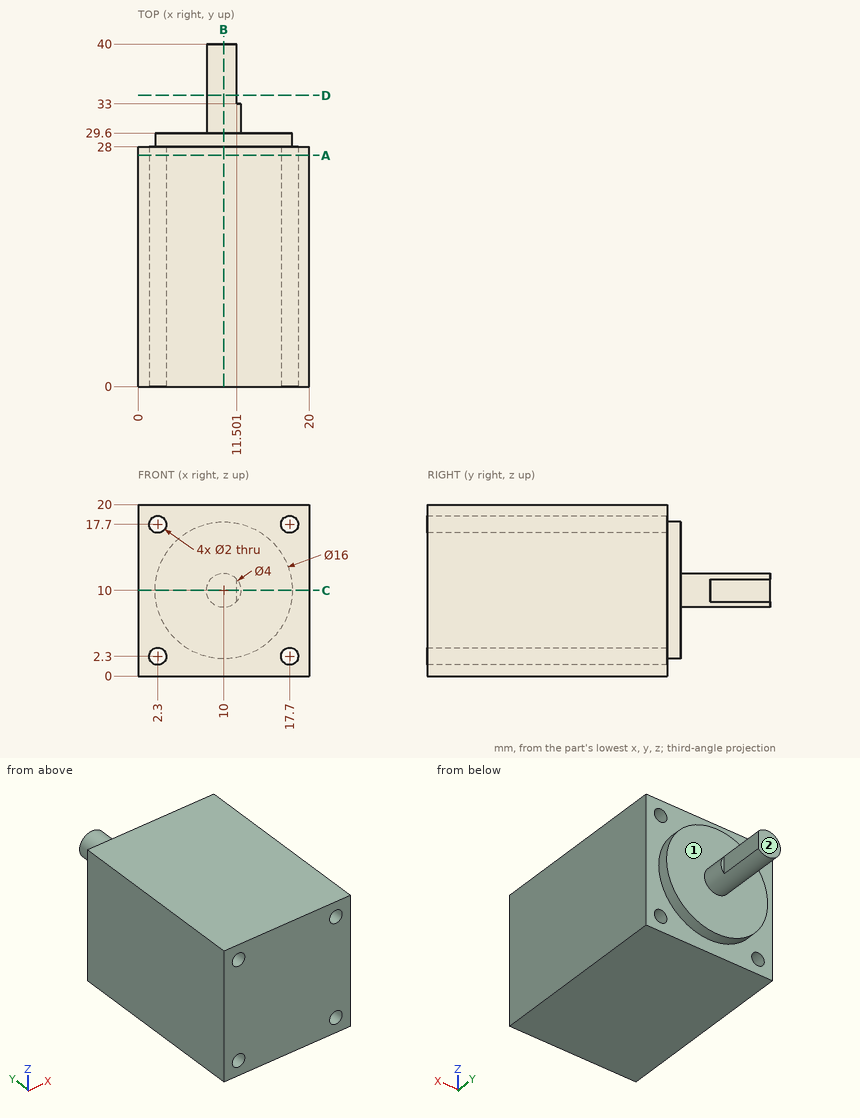
Answer from the drawing. Dimensions are ordinates in mm from the lowest x, y and z of the part. A direction names the side the tool comes from. Give positions to 0.01 mm unless a question says otherwise; leave off trailing zeros. Write each loop counter-clockwise with the first axis right and the second up, starting at its lowest first coordinate (ties: lowest second). Pieces come first, ordered by that corner, then holes. Notation, with made-up numbers: (72.25, 18) -> (95.25, 18) arc R11 cw to (95.25, 27) -> close; hole circle Ø6 at (-25, 42). An arc over 180 degrees is marked (long way). Use a Markdown table: item, result.
(1) Find the intervals of material crossed by probe 1 along X at (y, z) = (13.25, 2.3); probe 2 along Z at (x, y) = (17.25, 3.5); probe 3 along Y at (x, z) = (5.5, 17), in increasing order. Write a range as from..to.
Return value:
| item | result |
|---|---|
| probe 1 | 0..1.3, 3.3..16.7, 18.7..20 |
| probe 2 | 0..1.41, 3.19..16.81, 18.59..20 |
| probe 3 | 0..28 |
(2) Section A-A, the plane y = 27 is taken. Determine the outline of the cut face in (x, z), then the cut area to 3 significant figures.
Return value:
| item | result |
|---|---|
| outline | (0, 0) -> (20, 0) -> (20, 20) -> (0, 20) -> close; hole circle Ø2 at (2.3, 2.3); hole circle Ø2 at (2.3, 17.7); hole circle Ø2 at (17.7, 2.3); hole circle Ø2 at (17.7, 17.7) |
| area | 387 mm2 |
(3) Section D-D, the plane y = 34 is taken. Determine the outline of the cut face in (x, z), then the cut area to 3 significant figures.
Return value:
| item | result |
|---|---|
| outline | (11.5, 8.68) -> (11.5, 11.32) arc R2 ccw (long way) to start |
| area | 11.7 mm2 |
(4) Section C-C, the plane z = 10 is taken. Determine the outline of the cut face in (x, y).
Return value:
| item | result |
|---|---|
| outline | (0, 0) -> (20, 0) -> (20, 28) -> (18, 28) -> (18, 29.6) -> (12, 29.6) -> (12, 33) -> (11.5, 33) -> (11.5, 40) -> (8, 40) -> (8, 29.6) -> (2, 29.6) -> (2, 28) -> (0, 28) -> close |
(5) For the marked faces 1 and 2, determine the directions among +Z, -Z, +X, -X, +Y, -Y from which every point of the face is accessible in a straight line to the end or side of a thin tool.
Return value:
| item | result |
|---|---|
| face 1 | +Y |
| face 2 | +Z, -Z, +X, -X, +Y |
(6) Flat-ended cylindrical pins translate along their axes: P1, Ø1.8, axis at x = 2.3, z = 2.3, coming from the +Y side; P2, Ø3, axis at x = 15, z = 9, coming from the +Y side; P3, Ø2, axis at x = 2, z = 17, coming from the +Y side; P4, Ø3, axis at y = 36.5, z = 10.5, coming from the +X side. Find the tip coordinate at first contact, or state that the pin passes through.
Return value:
| item | result |
|---|---|
| P1 | through |
| P2 | y = 29.6 |
| P3 | y = 28 |
| P4 | x = 11.5 |
(7) Section B-B, the plane x = 10 is taken. Determine the outline of the cut face in (y, z), then the cut area to 3 significant figures.
Return value:
| item | result |
|---|---|
| outline | (0, 0) -> (28, 0) -> (28, 2) -> (29.6, 2) -> (29.6, 8) -> (40, 8) -> (40, 12) -> (29.6, 12) -> (29.6, 18) -> (28, 18) -> (28, 20) -> (0, 20) -> close |
| area | 627 mm2 |
